The model under review builds one solid part; all positions refer to its coordinate system, in mm. Face numbers are marked on the shaded views. A direction names the side the tool comes from. Coordinates: 2 decimals unless noted, no trailing zeros. Loops run counter-clockwise (first coordinate to the right, second up) from the corner with the lowest first, then second, coordinate; pieces in that order, holes last. Notation, with made-up numbers: M -8,65.5 L 28,65.5 A36 cw 28,103.5 Z; hole C -26,-33 d3. An arc over 180 degrees is marked long. Use one line per item in the form item = value.
Autodesk Inventor part; units mm, degrees
ref_plane "YZ Plane" through (0, 0, 0) normal (1, 0, 0) x (0, 1, 0)
ref_plane "XZ Plane" through (0, 0, 0) normal (0, 1, 0) x (-1, 0, 0)
ref_plane "XY Plane" through (0, 0, 0) normal (0, 0, 1) x (1, 0, 0)
sketch "Sketch1" plane through (0, 0, 0) normal (0, 1, 0) x (-1, 0, 0)
  circle A0 centre (0, 0) radius 22.225
  dimension "d0" = 44.45
extrude "Extrusion1" add sketch "Sketch1" along normal blind 3.175
fillet "Fillet1" radius 1.27 1 edges at (22.225, 0, 0)
sketch "Sketch2" plane through (0, 3.175, 0) normal (0, 1, 0) x (1, 0, 0)
  circle A0 centre (0, 0) radius 19.05
  dimension "d4" = 38.1
extrude "Extrusion2" add sketch "Sketch2" along normal blind 63.5
sketch "Sketch3" plane through (0, 66.675, 0) normal (0, 1, 0) x (1, 0, 0)
  circle A0 centre (0, 0) radius 17.145
  dimension "d7" = 34.29
extrude "Extrusion3" add sketch "Sketch3" along normal blind 228.6
sketch "Sketch4" plane through (0, 295.275, 0) normal (0, 1, 0) x (1, 0, 0)
  circle A0 centre (0, 0) radius 12.065
  dimension "d10" = 24.13
extrude "Extrusion4" add sketch "Sketch4" along normal blind 12.7
sketch "Sketch5" plane through (0, 307.975, 0) normal (0, 1, 0) x (1, 0, 0)
  circle A0 centre (0, 0) radius 8.89
  dimension "d14" = 17.78
extrude "Extrusion5" add sketch "Sketch5" along normal blind 6.35
fillet "Fillet3" radius 3.175 1 edges at (-8.89, 314.325, 0)
properties part number "middle shaft"
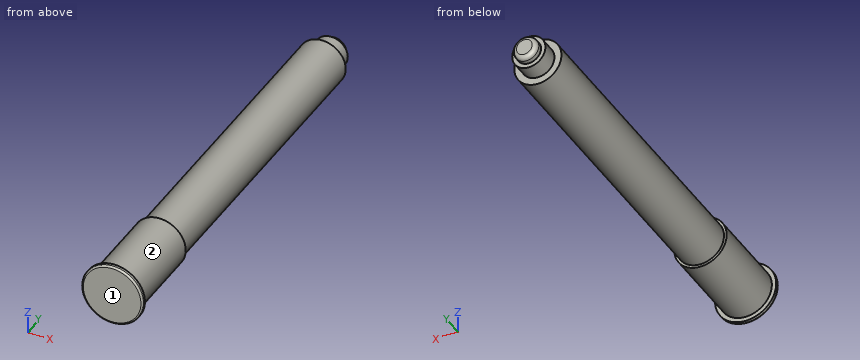
1. Add section B-B (z = 0). State the section outline as (x, y) points (3 decimals).
Response values:
outline = M -22.225,1.27 A1.27 ccw -20.955,0 L 20.955,0 A1.27 ccw 22.225,1.27 L 22.225,3.175 L 19.05,3.175 L 19.05,66.675 L 17.145,66.675 L 17.145,295.275 L 12.065,295.275 L 12.065,307.975 L 8.89,307.975 L 8.89,311.15 A3.175 ccw 5.715,314.325 L -5.715,314.325 A3.175 ccw -8.89,311.15 L -8.89,307.975 L -12.065,307.975 L -12.065,295.275 L -17.145,295.275 L -17.145,66.675 L -19.05,66.675 L -19.05,3.175 L -22.225,3.175 Z
2. Insertion check: P1, Ø10, axis at x = 12, z = 1, coming from the +Y side; P2, Ø12, axis at y = 143.5, z = -7, coming from the +X side; P3, Ø1.5, axis at x = 16, y = 178.5, coming from the -Z side. Each pin has a flat end and moves straight along its axis. Give the tip position at first contact, or say it passes through.
Response values:
P1 = 314.03
P2 = 17.12
P3 = -7.84
3. Add section A-A (x = 0). State the section outline as (y, z) points (3 decimals).
Response values:
outline = M 0,-20.955 A1.27 ccw 1.27,-22.225 L 3.175,-22.225 L 3.175,-19.05 L 66.675,-19.05 L 66.675,-17.145 L 295.275,-17.145 L 295.275,-12.065 L 307.975,-12.065 L 307.975,-8.89 L 311.15,-8.89 A3.175 ccw 314.325,-5.715 L 314.325,5.715 A3.175 ccw 311.15,8.89 L 307.975,8.89 L 307.975,12.065 L 295.275,12.065 L 295.275,17.145 L 66.675,17.145 L 66.675,19.05 L 3.175,19.05 L 3.175,22.225 L 1.27,22.225 A1.27 ccw 0,20.955 Z
4. Machinability: for the marked faces 1 and 2, which of the approach directions +Z, -Z, +X, -X, +Y, -Y give a long, thin tool a straight path to every point of the face, cutting with its end or side? Answer none if there is none.
Response values:
face_1 = +Z, -Z, +X, -X, -Y
face_2 = +Y
5. Wall thickness on line 1 along Z through (x, y) = (-0.5, 66); line 2 along Y through (x, z) = (-10, 18.5) (3 decimals); line 3 along Y through (x, z) = (-16, 7.5) (3 decimals): over which ranges is each line inside the solid? List them lowest first. Write a range as from..to.
Response values:
line_1 = -19.04..19.04
line_2 = 0.002..3.175
line_3 = 0..66.675
6. Add section C-C (y = 145.5). State the section outline as (x, z) points (3 decimals), then the cut area to 3 significant figures.
Response values:
outline = C 0,0 d34.29
area = 923 mm^2
